Design review of the part shown in the three views and the two pictorial views. Dimensions are in mm from the part's minimum x, y and z. Round coordinates to 2 decimals unless told otherwise and drop trailing zeros. Loops run counter-clockwise (first coordinate to the right, second up) from the corner with the lowest first, then second, coordinate; pieces in that order, holes last. Notation, with made-up numbers: M 44.5,34 L 76.5,34 A14 cw 76.5,55 Z; hole C 37.5,36 d1. An arc over 180 degrees is marked long. One line per question, with ' | ' between items.
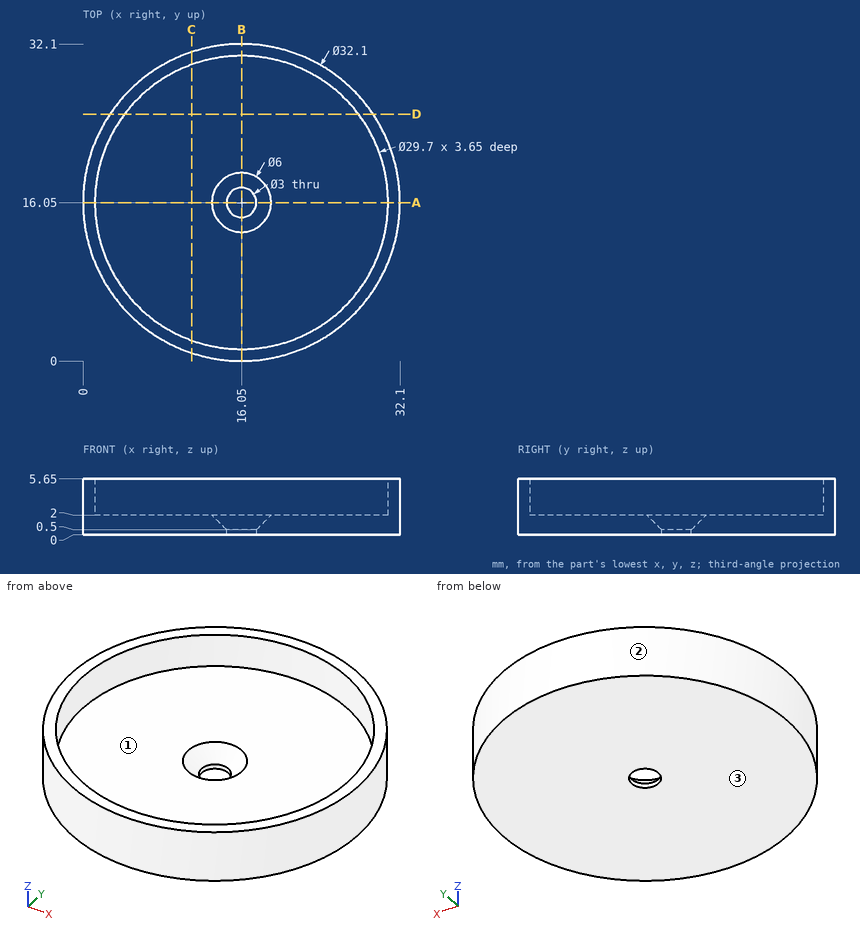
1) Add section A-A on y = 16.05. State the section outline as (x, z) points, then the cut area to 3 significant figures.
Output values:
outline: M 0,0 L 14.55,0 L 14.55,0.5 L 13.05,2 L 1.2,2 L 1.2,5.65 L 0,5.65 Z; M 17.55,0 L 32.1,0 L 32.1,5.65 L 30.9,5.65 L 30.9,2 L 19.05,2 L 17.55,0.5 Z | area: 64.7 mm²
2) Add section C-C on x = 11. State the section outline as (y, z) points, then the cut area to 3 significant figures.
Output values:
outline: M 0.82,0 L 31.28,0 L 31.28,5.65 L 30.01,5.65 L 30.01,2 L 2.09,2 L 2.09,5.65 L 0.82,5.65 Z | area: 70.2 mm²
3) For line 1 (Y direction, x = 16.05, z = 3.25); line 2 (Z direction, x = 11, y = 15.5); line 3 (Y direction, x = 13.5, z = 3.15), list the stretches that pass through material, from the lowest coordinate up.
Output values:
line 1: y = 0 to 1.2, 30.9 to 32.1 | line 2: z = 0 to 2 | line 3: y = 0.2 to 1.42, 30.68 to 31.9
4) Insertion check: P1, Ø9, axis at x = 19.5, y = 16.5, coming from the +Z side; P2, Ø1, axis at y = 15, z = 2, coming from the -X side; P3, Ø1.5, axis at y = 21.5, z = 5, coming from the +X side; P4, Ø5, axis at x = 16.05, y = 16.05, coming from the -Z side. Each pin has a flat end and moves straight along its axis. Give the tip position at first contact, or say it passes through.
Output values:
P1: stops at z = 2 | P2: stops at x = 0.01 | P3: stops at x = 31.4 | P4: stops at z = 0
5) Mouldability with a two-part tool opening along X and no side actions: class the marked faces 1, 2 and 3 as +X half, -X half, draft (parallel to the pull), parting line (faces both ways), or undercut.
Output values:
face 1: undercut | face 2: parting line | face 3: draft
6) Add section D-D on y = 25. State the section outline as (x, z) points.
Output values:
outline: M 2.73,0 L 29.37,0 L 29.37,5.65 L 27.9,5.65 L 27.9,2 L 4.2,2 L 4.2,5.65 L 2.73,5.65 Z
